```python
from build123d import *

# Parameters (mm, degrees)
SKETCH1_W           = 152.4
SKETCH1_H           = 152.4
BOSS_EXTRUDE1_DEPTH = 9.525
SKETCH2_W           = 139.7
SKETCH2_H           = 6.35
CUT_EXTRUDE1_DEPTH  = 10.525
LPATTERN1_COUNT     = 10
LPATTERN1_PITCH     = 12.7
SKETCH3_W           = 48.26
SKETCH3_H           = 6.35
SKETCH3_W_2         = 41.91
CUT_EXTRUDE2_DEPTH  = 9.525
LPATTERN2_COUNT     = 2
LPATTERN2_PITCH     = 12.7


with BuildPart() as part:
    # Sketch1 → Boss-Extrude1 (new body)
    with BuildSketch(Plane(origin=(0, 0, 0), x_dir=(1, 0, 0), z_dir=(0, 1, 0))):
        Rectangle(SKETCH1_W, SKETCH1_H)
    extrude(amount=BOSS_EXTRUDE1_DEPTH)

    # Sketch2 → Cut-Extrude1 (cut, through all)
    with BuildSketch(Plane.XZ):
        with Locations((0, 57.15)):
            Rectangle(SKETCH2_W, SKETCH2_H)
    cut_extrude1 = extrude(amount=-CUT_EXTRUDE1_DEPTH, mode=Mode.SUBTRACT)

    # LPattern1: Cut-Extrude1 ×10, 2 skipped
    with Locations(*[(0, 0, -i * LPATTERN1_PITCH) for i in range(1, LPATTERN1_COUNT) if i not in (4, 5)]):
        add(cut_extrude1, mode=Mode.SUBTRACT)

    # Sketch3 → Cut-Extrude2 (cut)
    with BuildSketch(Plane.XZ):
        with Locations((-45.72, 6.35)):
            Rectangle(SKETCH3_W, SKETCH3_H)
        with Locations((48.895, 6.35)):
            Rectangle(SKETCH3_W_2, SKETCH3_H)
    cut_extrude2 = extrude(amount=-CUT_EXTRUDE2_DEPTH, mode=Mode.SUBTRACT)

    # LPattern2: Cut-Extrude2 ×2
    with Locations(*[(0, 0, -i * LPATTERN2_PITCH) for i in range(1, LPATTERN2_COUNT)]):
        add(cut_extrude2, mode=Mode.SUBTRACT)


solid = part.part
```
Geometry check sheet. Reference: the model listing, model coordinates, mm. Coordinates: 2 decimals unless noted, no trailing zeros. Use CSV: the item, a comma, the result in double quotes. Start each with the question number.
Item 1: Mould release check, pull along Z, two halves, no side actions. Record for faces 1 (the flat face through (49, 5, -3.175)), 2 (the flat face through (69.85, 5, 57)), 3 (the flat face through (76.2, 5, 1)): released by +Z, released by -Z, zero draft, split by the parting line, or undercut.
Item 2: Cross-section at A-A, the plane y = 8. State how many separate pieces and enclosed holes the cut face has, plus the area to 3 significant figures.
Item 3: Thickness scan on line 1 (X direction, y = 2.5, z = 8.5); line 2 (X direction, y = 8.5, z = -32.5). Record the ranges inside material, lowest first.
Answers:
1,face 1,"undercut"
1,face 2,"undercut"
1,face 3,"zero draft"
2,separate pieces,"1"
2,enclosed holes,"12"
2,area,"15,000 mm^2"
3,line 1,"-76.2 to -69.85, -21.59 to 27.94, 69.85 to 76.2"
3,line 2,"-76.2 to -69.85, 69.85 to 76.2"
